Could you check a few things on this model? Use its own coordinates, in mm. Face numbers are marked on the shaded views. A direction names the side the tool comes from. Round coordinates to 2 decimals unless told otherwise and drop trailing zeros. Write each loop counter-clockwise with the first axis right and the second up, starting at its lowest first coordinate (ties: lowest second). Pieces come first, ordered by that corner, then holes. Notation, with made-up numbers: (-4.5, 4.25) - (10.5, 4.25) arc R16 ccw to (10.5, 33.25) - close; hole circle Ø3 at (21.25, 8.25). An arc over 180 degrees is marked (long way). Put each result on its own line as item: value.
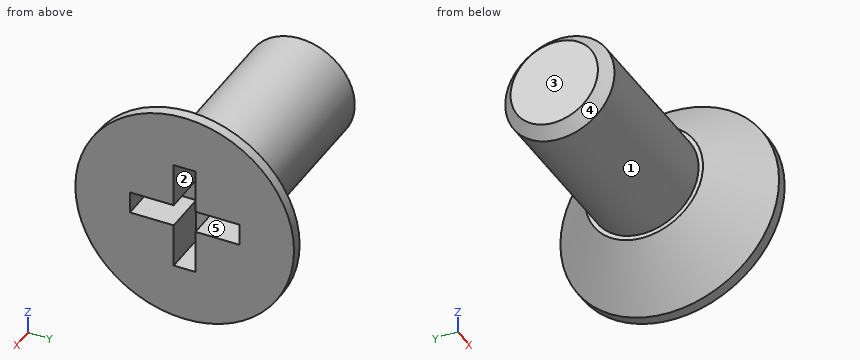
from build123d import *

# Parameters (mm, degrees)
F0_R     = 5
F1_DEPTH = 2.8
F2_R     = 2.5
F3_DEPTH = 8
F4_SIZE  = 2.3
F5_SIZE  = 0.5
F7_DEPTH = 2


with BuildPart() as f1:
    # F0 (on Right) → F1 (new body)
    with BuildSketch(Plane.YZ):
        Circle(F0_R)
    extrude(amount=-F1_DEPTH)

    # F2 (on face) → F3 (join)
    with BuildSketch(Plane(origin=(-2.8, 0, 0), x_dir=(0, -1, 0), z_dir=(-1, 0, 0))):
        Circle(F2_R)
    extrude(amount=F3_DEPTH)

    # F4
    f4_edges = [f1.edges().sort_by_distance(p)[0] for p in [
        (-2.8, -5, 0),
    ]]
    chamfer(f4_edges, length=F4_SIZE)

    # F5
    f5_edges = [f1.edges().sort_by_distance(p)[0] for p in [
        (-10.8, 2.5, 0),
    ]]
    chamfer(f5_edges, length=F5_SIZE)

    # F6 (on face) → F7 (cut)
    with BuildSketch(Plane.YZ):
        Polygon((0.5, 2.5), (0, 2.5), (-0.5, 2.5), (-0.5, 0.5), (-2.5, 0.5), (-2.5, 0), (-2.5, -0.5), (-0.5, -0.5), (-0.5, -2.5), (0, -2.5), (0.5, -2.5), (0.5, -0.5), (2.5, -0.5), (2.5, 0), (2.5, 0.5), (0.5, 0.5), align=None)
    extrude(amount=-F7_DEPTH, mode=Mode.SUBTRACT)


solid = f1.part
(1) Imagine slicing it at A-A, the plane x = -1.5. List the corners of the cut face in (y, z) for me, then the cut area to 3 significant figures.
Values found:
outline: circle Ø8 at (0, 0); hole (-2.5, -0.5) - (-0.5, -0.5) - (-0.5, -2.5) - (0.5, -2.5) - (0.5, -0.5) - (2.5, -0.5) - (2.5, 0.5) - (0.5, 0.5) - (0.5, 2.5) - (-0.5, 2.5) - (-0.5, 0.5) - (-2.5, 0.5) - close
area: 41.3 mm^2
(2) Please list where these lines run through material, in increasing order: probe 1 along X at (y, z) = (1.75, 2); probe 2 along Z at (x, y) = (-6.75, 1.75); probe 3 along Z at (x, y) = (-1.5, 0.75). Write a range as from..to.
Values found:
probe 1: x = -2.8..0
probe 2: z = -1.79..1.79
probe 3: z = -3.93..-0.5, 0.5..3.93
(3) Imagine slicing it at B-B, the plane z = 0. List the corners of the cut face in (x, y) for me.
Values found:
outline: (-10.8, -2) - (-10.3, -2.5) - (-2.8, -2.5) - (-2.8, -2.7) - (-0.5, -5) - (0, -5) - (0, -2.5) - (-2, -2.5) - (-2, 2.5) - (0, 2.5) - (0, 5) - (-0.5, 5) - (-2.8, 2.7) - (-2.8, 2.5) - (-10.3, 2.5) - (-10.8, 2) - close
(4) If we mould it in two halves opening along Y, with no side actions, what happens to the marked faces 1, 2 and 3? For each: pulls with the +Y half, pulls with the -Y half, needs draft (parallel to the pull), parting line crosses it, or undercut.
Values found:
face 1: parting line crosses it
face 2: undercut
face 3: needs draft
(5) For the marked faces 4 and 5, which set-ups out of +Z, -Z, +X, -X, +Y, -Y let a thin tool reach every point of the face, with its end or its side?
Values found:
face 4: -X
face 5: +X
(6) I'm going to push flat-ended pins straight in: pin 1 (2 mm diameter, centred on y = -0.5, z = -0.5, fed in from +X); pin 2 (1 mm diameter, centred on x = -1.5, z = -1.5, fed in from -Y); pin 3 (2 mm diameter, centred on x = -1, y = 1, fed in from +Z); pin 4 (0.6 mm diameter, centred on x = -1, y = -1.5, fed in from +Z). Where does each tip first touch, or does it pass through?
Values found:
pin 1: stops at x = 0
pin 2: stops at y = -4.27
pin 3: stops at z = 5
pin 4: stops at z = 4.57
(7) Imagine slicing it at D-D, the plane x = -9.25. List the corners of the cut face in (y, z) for me.
Values found:
outline: circle Ø5 at (0, 0)
